from build123d import *

# Parameters (mm, degrees)
SCHIZZO1_R                   = 125
SCHIZZO1_R_2                 = 101
ESTRUSIONE_ESTRUSIONE1_DEPTH = 80
RACCORDO1_R                  = 2
SCHIZZO3_R                   = 101
SCHIZZO3_R_2                 = 87
ESTRUSIONE_ESTRUSIONE2_DEPTH = 8.7
RACCORDO2_R                  = 1.5
SCHIZZO14_W                  = 10
SCHIZZO14_H                  = 35
TAGLIO_ESTRUSIONE1_DEPTH     = 71.3


with BuildPart() as part:
    # Schizzo1 → Estrusione-Estrusione1 (new body)
    with BuildSketch(Plane.XY):
        Circle(SCHIZZO1_R)
        Circle(SCHIZZO1_R_2, mode=Mode.SUBTRACT)
    extrude(amount=ESTRUSIONE_ESTRUSIONE1_DEPTH)

    # Raccordo1
    raccordo1_edges = [part.edges().sort_by_distance(p)[0] for p in [
        (-125, 0, 0),
        (-125, 0, 80),
    ]]
    fillet(raccordo1_edges, radius=RACCORDO1_R)

    # Schizzo3 → Estrusione-Estrusione2 (add)
    with BuildSketch(Plane.XY):
        Circle(SCHIZZO3_R)
        Circle(SCHIZZO3_R_2, mode=Mode.SUBTRACT)
    extrude(amount=ESTRUSIONE_ESTRUSIONE2_DEPTH)

    # Raccordo2
    raccordo2_edges = [part.edges().sort_by_distance(p)[0] for p in [
        (-87, 0, 0),
        (-87, 0, 8.7),
        (-101, 0, 80),
    ]]
    fillet(raccordo2_edges, radius=RACCORDO2_R)

    # Schizzo14 → Taglio-Estrusione1 (cut)
    with BuildSketch(Plane.XY.offset(80)):
        with Locations((0, 95)):
            Rectangle(SCHIZZO14_W, SCHIZZO14_H)
    extrude(amount=-TAGLIO_ESTRUSIONE1_DEPTH, mode=Mode.SUBTRACT)


solid = part.part
Source: CAD feature listing. Evaluate the final solid. Frame: model axes, mm. A direction names the side the tool comes from. Give positions to 0.01 mm unless a question says otherwise; leave off trailing zeros. Order: outer loops, then holes, each group sorted by start corner. A loop starts at its lowest first (then second) coordinate and runs counter-clockwise, first axis right, second up. Notation, with made-up numbers: (-20.75, 72.5) -> (14.25, 72.5) arc R8 ccw to (14.25, 81.5) -> close; hole circle Ø3 at (-25, 23). An arc over 180 degrees is marked (long way). Use a Markdown table: item, result.
1) Contact query for flat-ended pins moving along their axis: P1, Ø6, axis at x = 36.5, z = 53.5, coming from the +Y side; P2, Ø8, axis at x = 49.5, z = 56, coming from the -Y side; P3, Ø6, axis at y = 92.5, z = 64, coming from the +X side; P4, Ø3, axis at x = -79, y = 94.5, coming from the +Z side. Output: stop coordinate, or through.
Answer list:
| item | result |
|---|---|
| P1 | y = 120.43 |
| P2 | y = -116.42 |
| P3 | x = 87.26 |
| P4 | z = 80 |
2) Section query B-B, the plane z = 45.5. Return the cut outline in (x, y), then the cut area to 3 significant figures.
Answer list:
| item | result |
|---|---|
| outline | circle Ø250 at (0, 0); hole (-5, 100.88) arc R101 ccw (long way) to (5, 100.88) -> (5, 112.5) -> (-5, 112.5) -> close |
| area | 16,900 mm² |
3) Reachability of faces 5 (the cylindrical face through (-11.33, 86.26, 4.31)), 6 (the flat face through (0, 112.5, 45)) from +Z, -Z, +X, -X, +Y, -Y: full face, straight path, thin tool, end or side. Return the list, or none.
Answer list:
| item | result |
|---|---|
| face 5 | +Z, -Z |
| face 6 | +Z |
4) Mould query, pull axis Y, two halves, no side actions, for faces 1 (the flat face through (-92, 46, 80)), 2 (the cylindrical face through (-124.88, 5.5, 39.47)), 3 (the flat face through (5, 107, 45)), 4 (the flat face through (7, -89, 8.7)). Classes: +Y half, -Y half, draft (parallel to the pull), parting line (faces both ways), or undercut.
Answer list:
| item | result |
|---|---|
| face 1 | draft |
| face 2 | parting line |
| face 3 | undercut |
| face 4 | undercut |
5) Section query A-A, the plane x = 0. Return the cut outline in (y, z), then the cut area to 3 significant figures.
Answer list:
| item | result |
|---|---|
| outline | (-125, 2) arc R2 ccw to (-123, 0) -> (-88.5, 0) arc R1.5 ccw to (-87, 1.5) -> (-87, 7.2) arc R1.5 ccw to (-88.5, 8.7) -> (-101, 8.7) -> (-101, 78.5) arc R1.5 ccw to (-102.5, 80) -> (-123, 80) arc R2 ccw to (-125, 78) -> close; (87, 1.5) arc R1.5 ccw to (88.5, 0) -> (123, 0) arc R2 ccw to (125, 2) -> (125, 78) arc R2 ccw to (123, 80) -> (112.5, 80) -> (112.5, 8.7) -> (88.5, 8.7) arc R1.5 ccw to (87, 7.2) -> close |
| area | 3,260 mm² |
6) Ray query, line 1 along Y through (x, z) = (0, 5.2); line 2 along Y through (x, z) = (0, 39.5); line 3 along Z through (x, y) = (-92.5, -39). Return the intervals inside material, ascending. Write a range as [from, to].
Answer list:
| item | result |
|---|---|
| line 1 | [-125, -87], [87, 125] |
| line 2 | [-125, -101], [112.5, 125] |
| line 3 | [0, 8.7] |
